Read the model definition and answer for the solid it produces. Units are mm, in the model's axes. Face numbers are marked on the shaded views. A direction names the side the tool comes from. Give positions to 0.01 mm unless a question says otherwise; leave off trailing zeros. Order: outer loops, then holes, each group sorted by start corner. A loop starts at its lowest first (then second) coordinate and runs counter-clockwise, first axis right, second up. Notation, with made-up numbers: (4, 50) - (37, 50) arc R25 cw to (37, 77) - close; hole circle Ø5 at (85, 73). An arc over 180 degrees is marked (long way). Write each question's results on one line, items separated by ' | '.
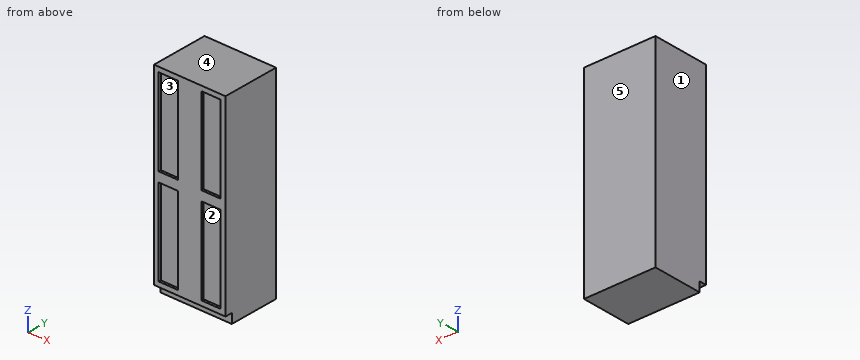
from build123d import *

# Parameters (mm, degrees)
F0_W     = 762
F0_H     = 609.6
F1_DEPTH = 2133.6
F2_W     = 762
F2_H     = 101.6
F3_DEPTH = 76.2
F4_W     = 203.2
F4_H     = 914.4
F5_DEPTH = 25.4


with BuildPart() as f1:
    # F0 (on Top) → F1 (new body)
    with BuildSketch(Plane.XY):
        with Locations((76.2, 0)):
            Rectangle(F0_W, F0_H)
    extrude(amount=F1_DEPTH)

    # F2 (on face) → F3 (cut)
    with BuildSketch(Plane.XZ.offset(304.8)):
        with Locations((76.2, 50.8)):
            Rectangle(F2_W, F2_H)
    extrude(amount=-F3_DEPTH, mode=Mode.SUBTRACT)

    # F4 (on face) → F5 (cut)
    with BuildSketch(Plane.XZ.offset(304.8)):
        with Locations((-152.4, 1625.6)):
            Rectangle(F4_W, F4_H)
        with Locations((304.8, 1625.6)):
            Rectangle(F4_W, F4_H)
        with Locations((304.8, 609.6)):
            Rectangle(F4_W, F4_H)
        with Locations((-152.4, 609.6)):
            Rectangle(F4_W, F4_H)
    extrude(amount=-F5_DEPTH, mode=Mode.SUBTRACT)


solid = f1.part
(1) Section B-B (z = 323.5) is taken. Give the vertices of the cut face in (x, y), plus the area to 3 significant figures.
Conclusion:
outline: (-304.8, -304.8) - (-254, -304.8) - (-254, -279.4) - (-50.8, -279.4) - (-50.8, -304.8) - (203.2, -304.8) - (203.2, -279.4) - (406.4, -279.4) - (406.4, -304.8) - (457.2, -304.8) - (457.2, 304.8) - (-304.8, 304.8) - close | area: 454,000 mm^2
(2) Consider probe 1 along Y at (x, z) = (-209.5, 837); probe 2 along Z at (x, y) = (-120, -231). Determine where each line is inside the solid, lowest interval first. Write a range as [from, to].
Conclusion:
probe 1: [-279.4, 304.8] | probe 2: [101.6, 2133.6]
(3) For the marked faces 1 and 2, determine the directions among +Z, -Z, +X, -X, +Y, -Y from which every point of the face is accessible in a straight line to the end or side of a thin tool.
Conclusion:
face 1: +Z, -Z, -X, +Y, -Y | face 2: -Y
(4) The mould has two halves that part along Z. Classify the marked faces 3, 4 and 5: pulls with the +Z half, pulls with the -Z half, needs draft (parallel to the pull), parting line crosses it, or undercut.
Conclusion:
face 3: undercut | face 4: pulls with the +Z half | face 5: needs draft
(5) Each of these flat-tipped pins is pushed along its axis until it touches: pin 1 (1 mm diameter, centred on x = -116, z = 1242, fed in from -Y); pin 2 (12.5 mm diameter, centred on x = 259, y = -291, fed in from -Z). Where does it stop, or does it pass through?
Conclusion:
pin 1: y = -279.4 | pin 2: z = 101.6
(6) Section A-A (x = 328.5) is taken. Give the vertices of the cut face in (y, z).
Conclusion:
outline: (-304.8, 101.6) - (-228.6, 101.6) - (-228.6, 0) - (304.8, 0) - (304.8, 2133.6) - (-304.8, 2133.6) - (-304.8, 2082.8) - (-279.4, 2082.8) - (-279.4, 1168.4) - (-304.8, 1168.4) - (-304.8, 1066.8) - (-279.4, 1066.8) - (-279.4, 152.4) - (-304.8, 152.4) - close
